```python
from build123d import *

# Parameters (mm, degrees)
SKETCH4_W                                      = 120
SKETCH4_H                                      = 120
BOSS_EXTRUDE2_DEPTH                            = 2.5
FILLET1_R                                      = 5
F_3_1_3_1_DIAMETER_HOLE1_D                     = 3.1
SKETCH8_R                                      = 11.1
CUT_EXTRUDE1_DEPTH                             = 10
SKETCH10_R                                     = 1
BOSS_EXTRUDE3_DEPTH                            = 16.499995
SKETCH11_R                                     = 1
BOSS_EXTRUDE4_DEPTH                            = 8
CSK_FOR_M2_5_FLAT_HEAD_MACHINE_SCREW2_AT_COUNT = 2
CSK_FOR_M2_5_FLAT_HEAD_MACHINE_SCREW2_AT_PITCH = 110
CSK_FOR_M2_5_FLAT_HEAD_MACHINE_SCREW_2_COUNT   = 2
CSK_FOR_M2_5_FLAT_HEAD_MACHINE_SCREW_2_PITCH   = 155.563491861
CSK_FOR_M2_5_FLAT_HEAD_MACHINE_SCREW_3_COUNT   = 2
CSK_FOR_M2_5_FLAT_HEAD_MACHINE_SCREW_3_PITCH   = 110


with BuildPart() as part:
    # Sketch4 → Boss-Extrude2 (new body)
    with BuildSketch(Plane.XY):
        with Locations((26, 26)):
            Rectangle(SKETCH4_W, SKETCH4_H)
        with BuildLine():
            Line((30.05, 64.884462408), (30.05, 44.884462408))
            ThreePointArc((30.05, 44.884462408), (26, 40.834462408), (21.95, 44.884462408))
            Line((21.95, 44.884462408), (21.95, 64.884462408))
            ThreePointArc((21.95, 64.884462408), (26, 68.934462408), (30.05, 64.884462408))
        make_face(mode=Mode.SUBTRACT)
    extrude(amount=BOSS_EXTRUDE2_DEPTH)

    # Fillet1
    fillet1_edges = [part.edges().sort_by_distance(p)[0] for p in [
        (-34, -34, 1.25),
        (-34, 86, 1.25),
        (86, 86, 1.25),
        (86, -34, 1.25),
    ]]
    fillet(fillet1_edges, radius=FILLET1_R)

    # Ø3.1 (3.1) Diameter Hole1 (through all)
    with Locations(Plane.XY.offset(2.5)):
        with Locations((-15.5, -15.5), (-15.5, 15.5), (15.5, 15.5), (15.5, -15.5), (36.5, -15.5), (36.5, 15.5), (67.5, -15.5), (67.5, 15.5)):
            Hole(F_3_1_3_1_DIAMETER_HOLE1_D / 2)

    # Sketch8 → Cut-Extrude1 (cut)
    with BuildSketch(Plane.XY.offset(2.5)):
        Circle(SKETCH8_R)
        with Locations((52, 0)):
            Circle(SKETCH8_R)
    extrude(amount=-CUT_EXTRUDE1_DEPTH, mode=Mode.SUBTRACT)

    # Sketch10 → Boss-Extrude3 (add)
    with BuildSketch(Plane.XY.offset(2.5)):
        with BuildLine():
            Line((-8.968535214, 38.85), (0.531464786, 38.85))
            ThreePointArc((0.531464786, 38.85), (6.531464786, 32.85), (0.531464786, 26.85))
            Line((0.531464786, 26.85), (-8.968535214, 26.85))
            ThreePointArc((-8.968535214, 26.85), (-14.968535214, 32.85), (-8.968535214, 38.85))
        make_face()
        with Locations((0.531464786, 32.85)):
            Circle(SKETCH10_R, mode=Mode.SUBTRACT)
        with Locations((-8.968535214, 32.85)):
            Circle(SKETCH10_R, mode=Mode.SUBTRACT)
    extrude(amount=BOSS_EXTRUDE3_DEPTH)

    # Sketch11 → Boss-Extrude4 (add)
    with BuildSketch(Plane.XY.offset(2.5)):
        with BuildLine():
            Line((-23.36906728, 57.461556068), (-14.085288007, 55.446254003))
            ThreePointArc((-14.085288007, 55.446254003), (-9.494670823, 48.309992105), (-16.63093272, 43.719374921))
            Line((-16.63093272, 43.719374921), (-25.914711993, 45.734676986))
            ThreePointArc((-25.914711993, 45.734676986), (-30.505329177, 52.870938884), (-23.36906728, 57.461556068))
        make_face()
        with Locations((-15.358110364, 49.582814462)):
            Circle(SKETCH11_R, mode=Mode.SUBTRACT)
        with Locations((-24.641889636, 51.598116527)):
            Circle(SKETCH11_R, mode=Mode.SUBTRACT)
    extrude(amount=BOSS_EXTRUDE4_DEPTH)

    # Sketch14 → CSK for M2.5 Flat Head Machine Screw2 (revolve, cut)
    with BuildSketch(Plane(origin=(81, 81, 2.5), x_dir=(0, -1, 0), z_dir=(1, 0, 0))):
        Polygon((0, 0), (0, 2.5), (1.45, 2.5), (1.45, 1.3), (2.75, 0), align=None)
    csk_for_m2_5_flat_head_machine_screw2 = revolve(axis=Axis((81, 81, 8.85), (0, 0, -1)), mode=Mode.SUBTRACT)

    # CSK for M2.5 Flat Head Machine Screw2 at: CSK for M2.5 Flat Head Machine Screw2 ×2
    with Locations(*[(0, -i * CSK_FOR_M2_5_FLAT_HEAD_MACHINE_SCREW2_AT_PITCH, 0) for i in range(1, CSK_FOR_M2_5_FLAT_HEAD_MACHINE_SCREW2_AT_COUNT)]):
        add(csk_for_m2_5_flat_head_machine_screw2, mode=Mode.SUBTRACT)

    # CSK for M2.5 Flat Head Machine Screw 2: CSK for M2.5 Flat Head Machine Screw2 ×2
    with Locations(*[Vector(-0.707106781, -0.707106781, 0) * (i * CSK_FOR_M2_5_FLAT_HEAD_MACHINE_SCREW_2_PITCH) for i in range(1, CSK_FOR_M2_5_FLAT_HEAD_MACHINE_SCREW_2_COUNT)]):
        add(csk_for_m2_5_flat_head_machine_screw2, mode=Mode.SUBTRACT)

    # CSK for M2.5 Flat Head Machine Screw 3: CSK for M2.5 Flat Head Machine Screw2 ×2
    with Locations(*[(-i * CSK_FOR_M2_5_FLAT_HEAD_MACHINE_SCREW_3_PITCH, 0, 0) for i in range(1, CSK_FOR_M2_5_FLAT_HEAD_MACHINE_SCREW_3_COUNT)]):
        add(csk_for_m2_5_flat_head_machine_screw2, mode=Mode.SUBTRACT)


solid = part.part
```
Work out the finished part from the listing and answer in its coordinate system (mm). A direction names the side the tool comes from. Round coordinates to 2 decimals unless told otherwise and drop trailing zeros. Order: outer loops, then holes, each group sorted by start corner. A loop starts at its lowest first (then second) coordinate and runs counter-clockwise, first axis right, second up.
Q1. Find the intervals of material crossed by line 1 along X through (y, z) = (-29, 0.8); line 2 along Y through (x, z) = (15.5, 0.85); line 3 along X through (y, z) = (32.5, 14.5), in increasing order.
Solution:
line 1: x = -34 to -30.45, -27.55 to 79.55, 82.45 to 86
line 2: y = -34 to -17.05, -13.95 to 13.95, 17.05 to 86
line 3: x = -14.96 to -9.91, -8.03 to -0.41, 1.47 to 6.52
Q2. A cutting plane is placed at A-A, the plane x = 52. Determine the outline of the cut face in (y, z), then the cut area to 4 significant figures.
Solution:
outline: (-34, 0) - (-11.1, 0) - (-11.1, 2.5) - (-34, 2.5) - close; (11.1, 0) - (86, 0) - (86, 2.5) - (11.1, 2.5) - close
area: 244.5 mm2
Q3. A cutting plane is placed at B-B, the plane y = 0. Determine the outline of the cut face in (x, z).
Solution:
outline: (-34, 0) - (-11.1, 0) - (-11.1, 2.5) - (-34, 2.5) - close; (11.1, 0) - (40.9, 0) - (40.9, 2.5) - (11.1, 2.5) - close; (63.1, 0) - (86, 0) - (86, 2.5) - (63.1, 2.5) - close
Q4. A tool of negligible diameter and unlimited length cuts with its end or side. For faces 1 (the cylindrical face through (6.53, 32.98, 10.63)), 2 (the cylindrical face through (-14.967, 32.718, 10.634)), 3 (the cylindrical face through (-33, -32, 1)), 4 (the cylindrical face through (25.911, 68.933, 1.232)), from which of +Z, -Z, +X, -X, +Y, -Y can it reach the whole face along a straight path? Write none if from no direction.
Solution:
face 1: +Z, +X
face 2: +Z, -X
face 3: +Z, -Z, -X, -Y
face 4: +Z, -Z
Q5. A cutting plane is placed at C-C, the plane z = 12. Determine the outline of the cut face in (x, y), then the cut area to 3 significant figures.
Solution:
outline: (-8.97, 26.85) - (0.53, 26.85) arc R6 ccw to (0.53, 38.85) - (-8.97, 38.85) arc R6 ccw to start; hole circle Ø2 at (-8.97, 32.85); hole circle Ø2 at (0.53, 32.85)
area: 221 mm2
Q6. The mould has two halves that part along Y. Classify faces 5 (the cylindrical face through (-30.532, 52.742, 6.444)), 6 (the flat face through (-4, 38.85, 11)), 7 (the cylindrical face through (66.022, -15.034, 1.232)): pulls with the +Y half, pulls with the -Y half, needs draft (parallel to the pull), parting line crosses it, or undercut.
Solution:
face 5: parting line crosses it
face 6: pulls with the +Y half
face 7: undercut
Q7. A cutting plane is placed at D-D, the plane y = 15.5. Determine the outline of the cut face in (x, z), then the cut area to 3 significant figures.
Solution:
outline: (-34, 0) - (-17.05, 0) - (-17.05, 2.5) - (-34, 2.5) - close; (-13.95, 0) - (13.95, 0) - (13.95, 2.5) - (-13.95, 2.5) - close; (17.05, 0) - (34.95, 0) - (34.95, 2.5) - (17.05, 2.5) - close; (38.05, 0) - (65.95, 0) - (65.95, 2.5) - (38.05, 2.5) - close; (69.05, 0) - (86, 0) - (86, 2.5) - (69.05, 2.5) - close
area: 269 mm2
Q8. Given pin 1 Ø1 at (x, y) = (22, -10) entering from +Z; pin 2 Ø8 at (x, z) = (-15, 11.5) entering from -Y; pin 3 Ø5 at (x, z) = (-3, 12) entering from +Y; pin 4 Ø3.5 at (x, y) = (-29, -29) entering from -Z, each flat-ended and moving along its own axis, determine where each tip first touches the part or whether it passes through.
Solution:
pin 1: stops at z = 2.5
pin 2: stops at y = 27.2
pin 3: stops at y = 38.85
pin 4: stops at z = 0
